```python
from build123d import *

# Parameters (mm, degrees)
SKETCH001_R       = 2.1
POCKET_DEPTH      = 24.001
POCKET_DEPTH_BACK = -24.001
CHAMFER_SIZE      = 0.5


with BuildPart() as part:
    # Sketch → Revolution (revolve)
    with BuildSketch(Plane.XZ):
        Polygon((24, 0), (-24, 0), (-24, 3.5), (-17, 3.5), (-16.42265, 4.5), (-9.154701, 4.5), (-8.57735, 5.5), (-0.57735, 5.5), (0, 4.5), (14.92265, 4.5), (15.5, 3.5), (24, 3.5), align=None)
    revolve(axis=Axis((0, 0, 0), (1, 0, 0)))

    # Sketch001 → Pocket (cut, two sides)
    with BuildSketch(Plane.YZ) as pocket_sk:
        Circle(SKETCH001_R)
    extrude(amount=-POCKET_DEPTH, mode=Mode.SUBTRACT)
    extrude(pocket_sk.sketch, amount=-POCKET_DEPTH_BACK, mode=Mode.SUBTRACT)

    # Chamfer
    chamfer_edges = [part.edges().sort_by_distance(p)[0] for p in [
        (-24, 0, -3.5),
        (24, 0, -3.5),
    ]]
    chamfer(chamfer_edges, length=CHAMFER_SIZE)


solid = part.part
```
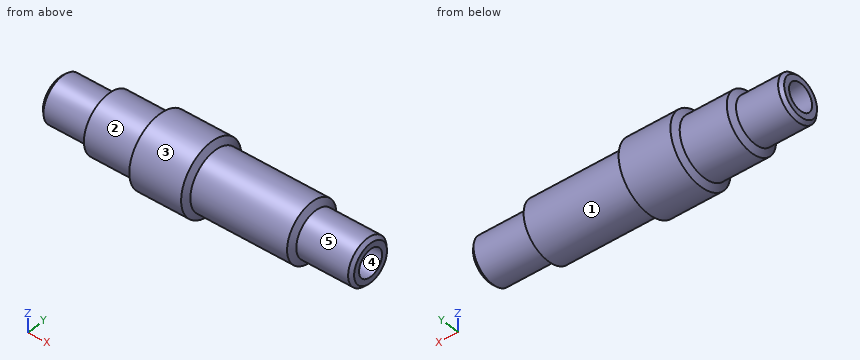
Input: part model. Units: mm. Frame: model coordinates. Face numbers are marked on the shaded views. A direction names the side the tool comes from. Coordinates: 2 decimals unless noted, no trailing zeros. Write each loop counter-clockwise with the first axis right and the second up, starting at its lowest first coordinate (ties: lowest second). Pieces come first, ordered by that corner, then holes.
1) Section C-C on x = 17. Output: boundary loops of the cut face in (y, z), and give its area (3 significant figures).
2) Pin query (flat end, axial travel): pin 1 Ø6 at (x, z) = (0.5, 4.5) entering from +Y; pin 2 Ø1 at (x, y) = (4.5, -0.5) entering from +Z; pin 3 Ø1 at (x, z) = (2, 0) entering from -Y. Return the tip coordinate at first contact, or that it passes through.
3) Section D-D on x = 5. Output: boundary loops of the cut face in (y, z), and give its area (3 significant figures).
4) Set-up query: the marked faces 1, 2 and 3. Return all of +Z, -Z, +X, -X, +Y, -Y with unobstructed straight access to the full face (end or side cutting, diameter ignored); none if empty.
5) Material intervals for line 1 along Z through (x, y) = (-6, 0); line 2 along Y through (x, z) = (9, 0), sorted ascending.
6) Section A-A on y = 0. Output: boundary loops of the cut face in (x, z).
7) Mould query, pull axis Y, two halves, no side actions, for the marked faces 4 and 5. Classes: pulls with the +Y half, pulls with the -Y half, needs draft (parallel to the pull), parting line crosses it, or undercut.
Check result:
1. outline: circle Ø7 at (0, 0); hole circle Ø4.2 at (0, 0)
1. area: 24.6 mm2
2. pin 1: stops at y = 5.23
2. pin 2: stops at z = 4.5
2. pin 3: stops at y = -4.5
3. outline: circle Ø9 at (0, 0); hole circle Ø4.2 at (0, 0)
3. area: 49.8 mm2
4. face 1: +X
4. face 2: -X
4. face 3: +X, -X
5. line 1: z = -5.5 to -2.1, 2.1 to 5.5
5. line 2: y = -4.5 to -2.1, 2.1 to 4.5
6. outline: (-24, -3) - (-23.5, -3.5) - (-17, -3.5) - (-16.42, -4.5) - (-9.15, -4.5) - (-8.58, -5.5) - (-0.58, -5.5) - (0, -4.5) - (14.92, -4.5) - (15.5, -3.5) - (23.5, -3.5) - (24, -3) - (24, -2.1) - (-24, -2.1) - close; (-24, 2.1) - (24, 2.1) - (24, 3) - (23.5, 3.5) - (15.5, 3.5) - (14.92, 4.5) - (0, 4.5) - (-0.58, 5.5) - (-8.58, 5.5) - (-9.15, 4.5) - (-16.42, 4.5) - (-17, 3.5) - (-23.5, 3.5) - (-24, 3) - close
7. face 4: undercut
7. face 5: parting line crosses it
